Geometry check sheet. Reference: the model listing, model coordinates, mm. A direction names the side the tool comes from. Coordinates: 2 decimals unless noted, no trailing zeros. Write each loop counter-clockwise with the first axis right and the second up, starting at its lowest first coordinate (ties: lowest second). Pieces come first, ordered by that corner, then holes. Notation, with made-up numbers: (19.25, 25.25) -> (37.25, 25.25) arc R16 ccw to (37.25, 36.25) -> close; hole circle Ø1 at (23, 87.5). An arc over 180 degrees is marked (long way). Use a Markdown table: item, result.
```python
from build123d import *

# Parameters (mm, degrees)
PAD_DEPTH       = 20
SKETCH006_R     = 10
POCKET_DEPTH    = 20.001
SKETCH005_R     = 11.05
POCKET001_DEPTH = 7
SKETCH002_R     = 2.25
POCKET002_DEPTH = 15.001
SKETCH003_R     = 5
POCKET003_DEPTH = 5


with BuildPart() as part:
    # Sketch → Pad (new body)
    with BuildSketch(Plane.XY):
        with BuildLine():
            Line((-35, 22), (35, 22))
            Line((35, 7), (35, 22))
            Line((20, 7), (35, 7))
            Line((20, 0), (20, 7))
            ThreePointArc((-20, 0), (0, -20), (20, 0))
            Line((-20, 0), (-20, 7))
            Line((-20, 7), (-35, 7))
            Line((-35, 7), (-35, 22))
        make_face()
    extrude(amount=PAD_DEPTH)

    # Sketch006 → Pocket (cut, through all)
    with BuildSketch(Plane(origin=(0, 0, 0), x_dir=(1, 0, 0), z_dir=(0, 0, -1))):
        Circle(SKETCH006_R)
    extrude(amount=-POCKET_DEPTH, mode=Mode.SUBTRACT)

    # Sketch005 → Pocket001 (cut)
    with BuildSketch(Plane.XY.offset(20)):
        Circle(SKETCH005_R)
    extrude(amount=-POCKET001_DEPTH, mode=Mode.SUBTRACT)

    # Sketch002 → Pocket002 (cut, through all)
    with BuildSketch(Plane.XZ.offset(-7)):
        with Locations((-27.5, 10)):
            Circle(SKETCH002_R)
        with Locations((27.5, 10)):
            Circle(SKETCH002_R)
    extrude(amount=-POCKET002_DEPTH, mode=Mode.SUBTRACT)

    # Sketch003 → Pocket003 (cut)
    with BuildSketch(Plane.XZ.offset(-7)):
        with Locations((-27.5, 10)):
            Circle(SKETCH003_R)
        with Locations((27.5, 10)):
            Circle(SKETCH003_R)
    extrude(amount=-POCKET003_DEPTH, mode=Mode.SUBTRACT)


solid = part.part
```
Item 1: Thickness scan on L1, parallel to X at y = 0, z = 2.75; L2, parallel to Z at x = -27.5, y = 8.75; L3, parallel to X at y = 1, z = 3.5. Record the ranges inside material, lowest first. Write a range as [from, to].
Answer block:
| item | result |
|---|---|
| L1 | x = [-20, -10], [10, 20] |
| L2 | z = [0, 5], [15, 20] |
| L3 | x = [-20, -9.95], [9.95, 20] |
Item 2: Mould release check, pull along Z, two halves, no side actions. Record for faces 1 (the cylindrical face through (0, -20, 10)), 2 (the cylindrical face through (22.505, 9.465, 10.22)), 3 (the flat face through (-7, 11, 20)): +Z half, -Z half, draft (parallel to the pull), parting line (faces both ways), or undercut.
Answer block:
| item | result |
|---|---|
| face 1 | draft |
| face 2 | undercut |
| face 3 | +Z half |
Item 3: Tool access check on faces 4 (the flat face through (-3, -10, 13)), 5 (the flat face through (20, 3, 10)), 6 (the cylindrical face through (-31.185, 9.465, 13.379)). Record the directions out of +Z, -Z, +X, -X, +Y, -Y that give a thin tool (end or side, any length) a straight path to the whole face; none if there is none.
Answer block:
| item | result |
|---|---|
| face 4 | +Z |
| face 5 | +Z, -Z, +X, -Y |
| face 6 | -Y |
Item 4: Section check B-B on x = -27.5. Record the boundary of the cut face in (y, z).
Answer block:
| item | result |
|---|---|
| outline | (7, 0) -> (22, 0) -> (22, 7.75) -> (12, 7.75) -> (12, 5) -> (7, 5) -> close; (7, 15) -> (12, 15) -> (12, 12.25) -> (22, 12.25) -> (22, 20) -> (7, 20) -> close |
Item 5: Section check A-A on z = 10. Record the boundary of the cut face in (x, y).
Answer block:
| item | result |
|---|---|
| outline | (-35, 7) -> (-32.5, 7) -> (-32.5, 12) -> (-29.75, 12) -> (-29.75, 22) -> (-35, 22) -> close; (-25.25, 12) -> (-22.5, 12) -> (-22.5, 7) -> (-20, 7) -> (-20, 0) arc R20 ccw to (20, 0) -> (20, 7) -> (22.5, 7) -> (22.5, 12) -> (25.25, 12) -> (25.25, 22) -> (-25.25, 22) -> close; (29.75, 12) -> (32.5, 12) -> (32.5, 7) -> (35, 7) -> (35, 22) -> (29.75, 22) -> close; hole circle Ø20 at (0, 0) |
Item 6: Depth check by flat-ended pin: P1, Ø9, axis at x = -27.5, z = 10, coming from the -Y side; P2, Ø5, axis at x = -18, z = 4.5, coming from the -Y side; P3, Ø12, axis at x = -29, z = 7, coming from the -Y side. Enter the tip coordinate at first touch or a pass-through.
Answer block:
| item | result |
|---|---|
| P1 | stops at y = 12 |
| P2 | stops at y = -12.64 |
| P3 | stops at y = 7 |
Item 7: Section check C-C on y = 16.5. Record the boundary of the cut face in (x, z), then the cut area to 3 significant figures.
Answer block:
| item | result |
|---|---|
| outline | (-35, 0) -> (35, 0) -> (35, 20) -> (-35, 20) -> close; hole circle Ø4.5 at (-27.5, 10); hole circle Ø4.5 at (27.5, 10) |
| area | 1,370 mm^2 |
Item 8: Section check D-D on z = 18. Record the boundary of the cut face in (x, y), then the cut area to 3 significant figures.
Answer block:
| item | result |
|---|---|
| outline | (-35, 7) -> (-20, 7) -> (-20, 0) arc R20 ccw to (20, 0) -> (20, 7) -> (35, 7) -> (35, 22) -> (-35, 22) -> close; hole circle Ø22.1 at (0, 0) |
| area | 1,570 mm^2 |
